Part model, mm, in its own coordinate system. A direction names the side the tool comes from. Round coordinates to 2 decimals unless told otherwise and drop trailing zeros. Loops run counter-clockwise (first coordinate to the right, second up) from the corner with the lowest first, then second, coordinate; pieces in that order, holes last. Notation, with made-up numbers: (0.5, 55) -> (42.5, 55) arc R11 cw to (42.5, 73) -> close; hole circle Ø9 at (73, 11). An arc over 180 degrees is marked (long way). Answer as CSV lines item,"result".
from build123d import *

# Parameters (mm, degrees)
SKETCH1_W                           = 600
SKETCH1_H                           = 600
BOSS_EXTRUDE1_DEPTH                 = 100
CUT_EXTRUDE1_DEPTH                  = 436.889894354
CHAMFER5_SIZE                       = 85
CUT_EXTRUDE2_DEPTH                  = 679.232998313
SKETCH9_R                           = 9.017
CUT_EXTRUDE5_DEPTH                  = 436.889894354
SKETCH12_R                          = 2.5
CUT_EXTRUDE7_DEPTH                  = 30
SKETCH14_W                          = 90
SKETCH14_H                          = 15
CUT_EXTRUDE8_DEPTH                  = 432.927077179
CHAMFER3_SIZE                       = 15
SKETCH15_W                          = 76.2
SKETCH15_H                          = 12.7
CUT_EXTRUDE9_DEPTH                  = 679.232998313
F_6_0MM_DOWEL_HOLE1_D               = 6
F_6_0MM_DOWEL_HOLE1_DEPTH           = 30
F_6_0MM_DOWEL_HOLE1_TIP             = 1.802581857
F_6_0MM_DOWEL_HOLE1_ON_FACE_2_D     = 6
F_6_0MM_DOWEL_HOLE1_ON_FACE_2_DEPTH = 30
F_6_0MM_DOWEL_HOLE1_ON_FACE_2_TIP   = 1.802581857
F_6_0MM_DOWEL_HOLE1_ON_FACE_3_D     = 6
F_6_0MM_DOWEL_HOLE1_ON_FACE_3_DEPTH = 30
F_6_0MM_DOWEL_HOLE1_ON_FACE_3_TIP   = 1.802581857
SKETCH23_R                          = 3.175
CUT_EXTRUDE10_DEPTH                 = 436.889894354
SKETCH24_R                          = 3
CUT_EXTRUDE11_DEPTH                 = 20
FILLET1_R                           = 80
F_5_0MM_DOWEL_HOLE1_D               = 5
F_5_0MM_DOWEL_HOLE1_DEPTH           = 28.497848452
F_5_0MM_DOWEL_HOLE1_TIP             = 1.502151548


with BuildPart() as part:
    # Sketch1 → Boss-Extrude1 (new body)
    with BuildSketch(Plane(origin=(0, 0, 0), x_dir=(1, 0, 0), z_dir=(0, 1, 0))):
        Rectangle(SKETCH1_W, SKETCH1_H)
    extrude(amount=BOSS_EXTRUDE1_DEPTH)

    # Sketch2 → Cut-Extrude1 (cut, through all)
    with BuildSketch(Plane(origin=(0, 100, 0), x_dir=(1, 0, 0), z_dir=(0, 1, 0))):
        Polygon((-300, -300), (-220, -300), (-215, -300), (-215, 74), (-220, 74), (-300, 74), (-300, 60), align=None)
        Polygon((300, -300), (220, -300), (215, -300), (215, 74), (220, 74), (300, 74), (300, 60), align=None)
    extrude(amount=-CUT_EXTRUDE1_DEPTH, mode=Mode.SUBTRACT)

    # Chamfer5
    chamfer5_edges = [part.edges().sort_by_distance(p)[0] for p in [
        (-215, 50, -74),
        (215, 50, -74),
    ]]
    chamfer(chamfer5_edges, length=CHAMFER5_SIZE - 0.0001)  # a hair under: the kernel refuses the full size

    # Sketch3 → Cut-Extrude2 (cut, through all)
    with BuildSketch(Plane.XY.offset(300)):
        Polygon((-35, 81), (-45, 81), (-65, 100), (-45, 100), (45, 100), (65, 100), (45, 81), (35, 81), (0, 81), align=None)
    extrude(amount=-CUT_EXTRUDE2_DEPTH, mode=Mode.SUBTRACT)

    # Sketch9 → Cut-Extrude5 (cut, through all)
    with BuildSketch(Plane(origin=(0, 100, 0), x_dir=(1, 0, 0), z_dir=(0, 1, 0))):
        with Locations(Location((275, 129, 0), (0, 0, 270))):
            Circle(SKETCH9_R)
        with Locations(Location((240, 129, 0), (0, 0, 270))):
            Circle(SKETCH9_R)
        with Locations(Location((240, 249, 0), (0, 0, 270))):
            Circle(SKETCH9_R)
        with Locations(Location((275, 249, 0), (0, 0, 270))):
            Circle(SKETCH9_R)
        with Locations(Location((-275, 129, 0), (0, 0, 90))):
            Circle(SKETCH9_R)
        with Locations(Location((-240, 249, 0), (0, 0, 90))):
            Circle(SKETCH9_R)
        with Locations(Location((-275, 249, 0), (0, 0, 90))):
            Circle(SKETCH9_R)
        with Locations(Location((-240, 129, 0), (0, 0, 90))):
            Circle(SKETCH9_R)
    extrude(amount=-CUT_EXTRUDE5_DEPTH, mode=Mode.SUBTRACT)

    # Sketch12 → Cut-Extrude7 (cut)
    with BuildSketch(Plane(origin=(0, 100, 0), x_dir=(1, 0, 0), z_dir=(0, 1, 0))):
        with Locations(Location((-100, -270, 0), (0, 0, 270))):
            Circle(SKETCH12_R)
        with Locations(Location((100, -270, 0), (0, 0, 270))):
            Circle(SKETCH12_R)
        with Locations(Location((100, -210, 0), (0, 0, 270))):
            Circle(SKETCH12_R)
        with Locations(Location((100, -150, 0), (0, 0, 270))):
            Circle(SKETCH12_R)
        with Locations(Location((100, -90, 0), (0, 0, 270))):
            Circle(SKETCH12_R)
        with Locations(Location((100, -30, 0), (0, 0, 270))):
            Circle(SKETCH12_R)
        with Locations(Location((100, 30, 0), (0, 0, 270))):
            Circle(SKETCH12_R)
        with Locations(Location((100, 90, 0), (0, 0, 270))):
            Circle(SKETCH12_R)
        with Locations(Location((100, 150, 0), (0, 0, 270))):
            Circle(SKETCH12_R)
        with Locations(Location((100, 210, 0), (0, 0, 270))):
            Circle(SKETCH12_R)
        with Locations(Location((100, 270, 0), (0, 0, 270))):
            Circle(SKETCH12_R)
        with Locations(Location((-100, -210, 0), (0, 0, 270))):
            Circle(SKETCH12_R)
        with Locations(Location((-100, -150, 0), (0, 0, 270))):
            Circle(SKETCH12_R)
        with Locations(Location((-100, -90, 0), (0, 0, 270))):
            Circle(SKETCH12_R)
        with Locations(Location((-100, -30, 0), (0, 0, 270))):
            Circle(SKETCH12_R)
        with Locations(Location((-100, 30, 0), (0, 0, 270))):
            Circle(SKETCH12_R)
        with Locations(Location((-100, 90, 0), (0, 0, 270))):
            Circle(SKETCH12_R)
        with Locations(Location((-100, 150, 0), (0, 0, 270))):
            Circle(SKETCH12_R)
        with Locations(Location((-100, 210, 0), (0, 0, 270))):
            Circle(SKETCH12_R)
        with Locations(Location((-100, 270, 0), (0, 0, 270))):
            Circle(SKETCH12_R)
    extrude(amount=-CUT_EXTRUDE7_DEPTH, mode=Mode.SUBTRACT)

    # Sketch14 → Cut-Extrude8 (cut, through all)
    with BuildSketch(Plane(origin=(0, 81, 0), x_dir=(1, 0, 0), z_dir=(0, 1, 0))):
        with Locations((0, -292.5)):
            Rectangle(SKETCH14_W, SKETCH14_H)
    extrude(amount=-CUT_EXTRUDE8_DEPTH, mode=Mode.SUBTRACT)

    # Chamfer3
    chamfer3_edges = [part.edges().sort_by_distance(p)[0] for p in [
        (45, 40.5, 300),
        (-45, 40.5, 300),
    ]]
    chamfer(chamfer3_edges, length=CHAMFER3_SIZE - 0.0001)  # a hair under: the kernel refuses the full size

    # Sketch15 → Cut-Extrude9 (cut, through all)
    with BuildSketch(Plane.ZY.offset(300)):
        with Locations((86.9, 5.65)):
            Rectangle(SKETCH15_W, SKETCH15_H)
        with Locations((-189.9, 5.65)):
            Rectangle(SKETCH15_W, SKETCH15_H)
    extrude(amount=-CUT_EXTRUDE9_DEPTH, mode=Mode.SUBTRACT)

    # Ø6.0mm Dowel Hole1
    with Locations(Plane(origin=(-30, 66, 285), x_dir=(1, 0, 0), z_dir=(0, 0, 1))):
        with Locations((0, 0), (60, 0), (60, -51), (0, -51)):
            Hole(F_6_0MM_DOWEL_HOLE1_D / 2, depth=F_6_0MM_DOWEL_HOLE1_DEPTH)
            with Locations((0, 0, -(F_6_0MM_DOWEL_HOLE1_DEPTH + F_6_0MM_DOWEL_HOLE1_TIP / 2))):  # 118° drill point
                Cone(0, F_6_0MM_DOWEL_HOLE1_D / 2, F_6_0MM_DOWEL_HOLE1_TIP, mode=Mode.SUBTRACT)

    # Ø6.0mm Dowel Hole1 on face 2
    with Locations(Plane(origin=(30, 66, -300), x_dir=(-1, 0, 0), z_dir=(0, 0, -1))):
        with Locations((0, 0), (60, 0), (60, -51), (0, -51), (145, 14), (115, 14), (-55, 14), (-85, 14), (145, -46), (115, -46), (-55, -46), (-85, -46)):
            Hole(F_6_0MM_DOWEL_HOLE1_ON_FACE_2_D / 2, depth=F_6_0MM_DOWEL_HOLE1_ON_FACE_2_DEPTH)
            with Locations((0, 0, -(F_6_0MM_DOWEL_HOLE1_ON_FACE_2_DEPTH + F_6_0MM_DOWEL_HOLE1_ON_FACE_2_TIP / 2))):  # 118° drill point
                Cone(0, F_6_0MM_DOWEL_HOLE1_ON_FACE_2_D / 2, F_6_0MM_DOWEL_HOLE1_ON_FACE_2_TIP, mode=Mode.SUBTRACT)

    # Ø6.0mm Dowel Hole1 on face 3
    with Locations(Plane(origin=(-85, 50, 300), x_dir=(1, 0, 0), z_dir=(0, 0, 1))):
        with Locations((0, 0), (-30, 0), (170, 0), (200, 0), (-30, -30), (0, -30), (170, -30), (200, -30)):
            Hole(F_6_0MM_DOWEL_HOLE1_ON_FACE_3_D / 2, depth=F_6_0MM_DOWEL_HOLE1_ON_FACE_3_DEPTH)
            with Locations((0, 0, -(F_6_0MM_DOWEL_HOLE1_ON_FACE_3_DEPTH + F_6_0MM_DOWEL_HOLE1_ON_FACE_3_TIP / 2))):  # 118° drill point
                Cone(0, F_6_0MM_DOWEL_HOLE1_ON_FACE_3_D / 2, F_6_0MM_DOWEL_HOLE1_ON_FACE_3_TIP, mode=Mode.SUBTRACT)

    # Sketch23 → Cut-Extrude10 (cut, through all)
    with BuildSketch(Plane(origin=(0, 100, 0), x_dir=(1, 0, 0), z_dir=(0, 1, 0))):
        with Locations(Location((-257.5, 189, 0), (0, 0, 270))):
            Circle(SKETCH23_R)
        with Locations(Location((257.5, 189, 0), (0, 0, 270))):
            Circle(SKETCH23_R)
    extrude(amount=-CUT_EXTRUDE10_DEPTH, mode=Mode.SUBTRACT)

    # Sketch24 → Cut-Extrude11 (cut)
    with BuildSketch(Plane(origin=(0, 100, 0), x_dir=(1, 0, 0), z_dir=(0, 1, 0))):
        with Locations(Location((255, 64, 0), (0, 0, 270))):
            Circle(SKETCH24_R)
        with Locations(Location((220, 39, 0), (0, 0, 270))):
            Circle(SKETCH24_R)
        with Locations(Location((-220, 39, 0), (0, 0, 90))):
            Circle(SKETCH24_R)
        with Locations(Location((-255, 64, 0), (0, 0, 90))):
            Circle(SKETCH24_R)
    extrude(amount=-CUT_EXTRUDE11_DEPTH, mode=Mode.SUBTRACT)

    # Fillet1
    fillet1_edges = [part.edges().sort_by_distance(p)[0] for p in [
        (-215, 50, 10.9999),
        (215, 50, 10.9999),
    ]]
    fillet(fillet1_edges, radius=FILLET1_R)

    # Ø5.0mm Dowel Hole1
    with Locations(Plane(origin=(0, 100, 0), x_dir=(1, 0, 0), z_dir=(0, 1, 0))):
        with Locations((-150, 270), (150, 270), (-150, 90), (150, 90), (-150, -90), (150, -90), (-150, -270), (150, -270), (150, 180), (-150, 180), (-150, 0), (150, 0), (150, -180), (-150, -180)):
            Hole(F_5_0MM_DOWEL_HOLE1_D / 2, depth=F_5_0MM_DOWEL_HOLE1_DEPTH)
            with Locations((0, 0, -(F_5_0MM_DOWEL_HOLE1_DEPTH + F_5_0MM_DOWEL_HOLE1_TIP / 2))):  # 118° drill point
                Cone(0, F_5_0MM_DOWEL_HOLE1_D / 2, F_5_0MM_DOWEL_HOLE1_TIP, mode=Mode.SUBTRACT)


solid = part.part
Q1. Saw through at B-B, the plane x = 73.5. Write the cut outline in (y, z).
Geometry results:
outline,"(0, -300) -> (100, -300) -> (100, 300) -> (0, 300) -> (0, 125) -> (12, 125) -> (12, 48.8) -> (0, 48.8) -> (0, -151.8) -> (12, -151.8) -> (12, -228) -> (0, -228) -> close"
Q2. Two-plate mould, pull along X, no slides. Class faces 5 (the face through (-3, 12, 86)), 6 (the face through (300, 49, -185)), 7 (the face through (-266.197, 50.7, -127.045)): pulls with the +X half, pulls with the -X half, needs draft (parallel to the pull), parting line crosses it, or undercut.
Geometry results:
face 5,"needs draft"
face 6,"pulls with the +X half"
face 7,"undercut"
Q3. Which spindle directions (+Z, -Z, +X, -X, +Y, -Y) get a long thin tool onto all of the face, cutting with end or side? Do faces 1 (the face through (-4, 12, -190)), 2 (the face through (52, 48, 292)), 3 (the face through (215, 51, 174)), 4 (the face through (-215, 51, 174)). Say none if no direction does.
Geometry results:
face 1,"+X, -X, -Y"
face 2,"+Z, +Y, -Y"
face 3,"+Z, +X, +Y, -Y"
face 4,"+Z, -X, +Y, -Y"
Q4. Drop flat-ended pins along their axis: P1, Ø4.5, axis at x = 150, z = 90, coming from the -Y side; P2, Ø4, axis at x = 20.5, y = 22.5, coming from the +Z side; P3, Ø5, axis at y = 66.5, z = 229.5, coming from the -X side. Give the stop position or say it passes through.
Geometry results:
P1,"y = 12"
P2,"z = 285"
P3,"x = -215"
Q5. Drill centre lines: line 1 along X through (y, z) = (80, -288); line 2 along Y through (x, z) = (115, 274); line 3 along X through (y, z) = (78, -90). Where is each one in solid material? Low to high.
Geometry results:
line 1,"-300 to -118, -112 to -88, -82 to 82, 88 to 112, 118 to 300"
line 2,"0 to 17, 23 to 47, 53 to 100"
line 3,"-300 to -152.5, -147.5 to -102.5, -97.5 to 97.5, 102.5 to 147.5, 152.5 to 300"
Q6. Saw through at A-A, the plane y = 32. Give the number of separate pieces and of enclosed holes in the cut face, then the cut area to 3 significant figures.
Geometry results:
separate pieces,"1"
enclosed holes,"10"
area,"300,000 mm2"
